```python
from build123d import *

# Parameters (mm, degrees)
BOSS_EXTRUDE1_DEPTH   = 3
F_6_CLEARANCE_HOLE2_D = 3.7973
SKETCH10_R            = 2.025
CUT_EXTRUDE1_DEPTH    = 10
F_4_CLEARANCE_HOLE3_D = 3.2639


with BuildPart() as part:
    # Sketch1 → Boss-Extrude1 (new body)
    with BuildSketch(Plane(origin=(0, 0, 0), x_dir=(0, 0, -1), z_dir=(1, 0, 0))):
        with BuildLine():
            Line((0, 0), (40, 0))
            Line((40, 0), (40, 52.5))
            ThreePointArc((40, 52.5), (35.606601718, 63.106601718), (25, 67.5))
            Line((25, 67.5), (15, 67.5))
            ThreePointArc((15, 67.5), (4.393398282, 63.106601718), (0, 52.5))
            Line((0, 52.5), (0, 0))
        make_face()
    extrude(amount=BOSS_EXTRUDE1_DEPTH)

    # #6 Clearance Hole2 (through all)
    with Locations(Plane(origin=(3, 0, 0), x_dir=(0, 0, -1), z_dir=(1, 0, 0))):
        with Locations((7.5, 5), (20, 5), (32.5, 5)):
            Hole(F_6_CLEARANCE_HOLE2_D / 2)

    # Sketch10 → Cut-Extrude1 (cut)
    with BuildSketch(Plane(origin=(3, 0, 0), x_dir=(0, 0, -1), z_dir=(1, 0, 0))):
        with Locations((20, 52.5)):
            Circle(SKETCH10_R)
    extrude(amount=-CUT_EXTRUDE1_DEPTH, mode=Mode.SUBTRACT)

    # #4 Clearance Hole3 (through all)
    with Locations(Plane(origin=(3, 0, 0), x_dir=(0, 0, -1), z_dir=(1, 0, 0))):
        with Locations((10, 52.5), (30, 52.5)):
            Hole(F_4_CLEARANCE_HOLE3_D / 2)


solid = part.part
```
Can you work these out from the model? Positions are in its coordinate system, mm. Coordinates: 2 decimals unless noted, no trailing zeros. Loops run counter-clockwise (first coordinate to the right, second up) from the corner with the lowest first, then second, coordinate; pieces in that order, holes last. Notation, with made-up numbers: (2, 44) -> (57, 44) arc R22 ccw to (57, 63) -> close; hole circle Ø4 at (-26, -33). An arc over 180 degrees is marked (long way). Answer as a JSON object with one key per item and string values.
1) Imagine slicing it at B-B (z = -20). Please give me the cut outline in (x, y) (3 decimals), then the cut area to 3 significant figures.
Results:
{"outline": "(0, 0) -> (3, 0) -> (3, 3.101) -> (0, 3.101) -> close; (0, 6.899) -> (3, 6.899) -> (3, 50.475) -> (0, 50.475) -> close; (0, 54.525) -> (3, 54.525) -> (3, 67.5) -> (0, 67.5) -> close", "area": "179 mm^2"}
2) Imagine slicing it at C-C (z = -7.5). Please give me the cut outline in (x, y), then the cut area to 3 significant figures.
Results:
{"outline": "(0, 0) -> (3, 0) -> (3, 3.1) -> (0, 3.1) -> close; (0, 6.9) -> (3, 6.9) -> (3, 65.49) -> (0, 65.49) -> close", "area": "185 mm^2"}
3) Thinking about a two-plate mould opening in Z: for faces 1 (the face through (1.5, 5.6, -5.7)), 2 (the face through (1.48, 62.99, -35.72)), 3 (the face through (1, 67.5, -20)), 4 (the face through (1.5, 5.6, -30.7)), which applies, pulls with the +Z half, pulls with the -Z half, needs draft (parallel to the pull), parting line crosses it, or undercut?
Results:
{"face 1": "undercut", "face 2": "pulls with the -Z half", "face 3": "needs draft", "face 4": "undercut"}
4) Imagine slicing it at A-A (x = 2.05). Please give me the cut outline in (y, z) (3 decimals).
Results:
{"outline": "(0, -40) -> (52.5, -40) arc R15 ccw to (67.5, -25) -> (67.5, -15) arc R15 ccw to (52.5, 0) -> (0, 0) -> close; hole circle Ø3.797 at (5, -32.5); hole circle Ø3.797 at (5, -20); hole circle Ø3.797 at (5, -7.5); hole circle Ø4.05 at (52.5, -20); hole circle Ø3.264 at (52.5, -30); hole circle Ø3.264 at (52.5, -10)"}
5) For P1, Ø6, axis at y = 17, z = -13.5, coming from the -X side, with a flat end and sliding along its axis, tell me the tip position at first contact or that it passes through.
Results:
{"P1": "stops at x = 0"}
6) If I drill on line 1 (Y direction, x = 1.9, z = -20) (3 decimals); line 2 (Y direction, x = 2.6, z = -8.5); line 3 (Y direction, x = 1.45, z = -32.5), over which ranges is the centre line in solid material (lowest first)?
Results:
{"line 1": "y = 0 to 3.101, 6.899 to 50.475, 54.525 to 67.5", "line 2": "y = 0 to 3.39, 6.61 to 51.86, 53.14 to 66.02", "line 3": "y = 0 to 3.1, 6.9 to 65.49"}
